Read the model definition and answer for the solid it produces. Units are mm, in the model's axes. Face numbers are marked on the shaded views. A direction names the side the tool comes from. Coordinates: 2 decimals unless noted, no trailing zeros. Order: outer loops, then holes, each group sorted by start corner. A loop starts at its lowest first (then second) coordinate and runs counter-clockwise, first axis right, second up. Notation, with made-up numbers: (89.5, -27.75) -> (135.5, -27.75) arc R18 cw to (135.5, -10.75) -> close; hole circle Ø5 at (-3.75, 21.5). An arc over 180 degrees is marked (long way). Use CSV: the item, a comma, the result in double quotes.
```python
from build123d import *

# Parameters (mm, degrees)
CROQUIS1_R              = 1.651
CROQUIS1_R_2            = 1.3208
SALIENTE_EXTRUIR1_DEPTH = 3.1242
CORTAR_EXTRUIR1_DEPTH   = 3.1242


with BuildPart() as part:
    # Croquis1 → Saliente-Extruir1 (new body)
    with BuildSketch(Plane.XY):
        with BuildLine():
            ThreePointArc((2.520278818, -2.298225244), (5.5245, -0.523415469), (8.528721182, -2.298225244))
            ThreePointArc((8.528721182, -2.298225244), (15.964986845, -3.467169905), (15.244404767, 4.025842847))
            ThreePointArc((15.244404767, 4.025842847), (7.556394525, 12.189930179), (4.7625, 23.0505))
            ThreePointArc((4.7625, 23.0505), (-0.866847253, 27.733445877), (-4.446941298, 21.345765609))
            ThreePointArc((-4.446941298, 21.345765609), (-3.013234987, 11.681947272), (-5.809588918, 2.321108456))
            ThreePointArc((-5.809588918, 2.321108456), (-3.960675565, -4.164949584), (2.520278818, -2.298225244))
        make_face()
        with Locations((-1.651, 0)):
            Circle(CROQUIS1_R, mode=Mode.SUBTRACT)
        Polygon((4.638514436, 4.7625), (3.464816339, 4.7625), (3.599843554, 6.647687651), align=None, mode=Mode.SUBTRACT)
        with Locations((0, 23.0505)):
            Circle(CROQUIS1_R_2, mode=Mode.SUBTRACT)
        with Locations((12.7, 0)):
            Circle(CROQUIS1_R, mode=Mode.SUBTRACT)
    extrude(amount=SALIENTE_EXTRUIR1_DEPTH)

    # Croquis2 → Cortar-Extruir1 (cut)
    with BuildSketch(Plane.XY.offset(3.1242)):
        with BuildLine():
            ThreePointArc((6.772401381, 2.38125), (7.178118311, 3.26217793), (7.753887726, 4.042645627))
            Line((7.753887726, 4.042645627), (2.361995667, 13.828929715))
            ThreePointArc((2.361995667, 13.828929715), (2.041810785, 13.746918232), (1.71670875, 13.687311946))
            Line((1.71670875, 13.687311946), (1.018825269, 3.943784893))
            ThreePointArc((1.018825269, 3.943784893), (1.834815442, 3.24507272), (2.473445986, 2.38125))
            Line((2.473445986, 2.38125), (6.772401381, 2.38125))
        make_face()
    extrude(amount=-CORTAR_EXTRUIR1_DEPTH, mode=Mode.SUBTRACT)


solid = part.part
```
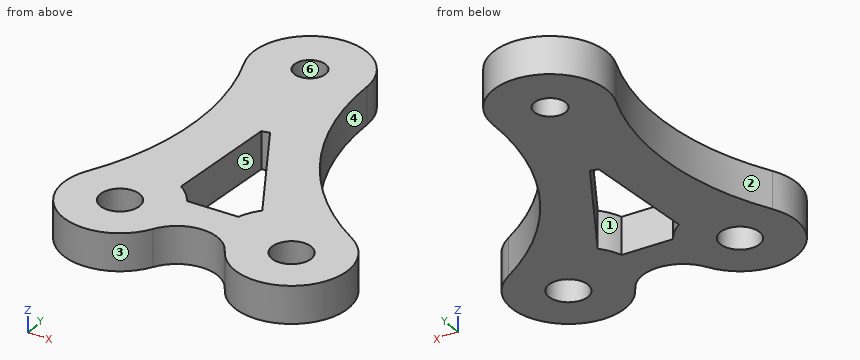
Item 1: The mould has two halves that part along Y. Classify the marked faces 3, 4, 5 and 6: +Y half, -Y half, draft (parallel to the pull), parting line (faces both ways), or undercut.
Return value:
face 3,"parting line"
face 4,"+Y half"
face 5,"undercut"
face 6,"undercut"
Item 2: A tool of negligible diameter and unlimited length cuts with its end or side. For the marked faces 1 and 2, from which of +Z, -Z, +X, -X, +Y, -Y can it reach the whole face along a straight path? Write none if from no direction.
Return value:
face 1,"+Z, -Z"
face 2,"+Z, -Z, -X"
Item 3: Find section D-D, the plane y = 20. Give the vertices of the cut face in (x, z), then the cut area to 3 significant figures.
Return value:
outline,"(-3.98, 0) -> (4.97, 0) -> (4.97, 3.12) -> (-3.98, 3.12) -> close"
area,"28.0 mm^2"
Item 4: Find section C-C, the plane z = 2.55. Give the vertices of the cut face in (x, y) (1 decimal), then the cut area to 3 significant figures.
Return value:
outline,"(-5.8, 2.3) arc R4.8 ccw to (2.5, -2.3) arc R3.4 cw to (8.5, -2.3) arc R4.8 ccw (long way) to (15.2, 4) arc R22.5 cw to (4.8, 23.1) arc R4.8 ccw (long way) to (-4.4, 21.3) arc R22.5 cw to start; hole circle Ø3.3 at (-1.7, 0); hole circle Ø2.6 at (0, 23.1); hole (1, 3.9) arc R4.8 cw to (2.5, 2.4) -> (6.8, 2.4) arc R4.8 cw to (7.8, 4) -> (2.4, 13.8) arc R4.8 cw to (1.7, 13.7) -> close; hole circle Ø3.3 at (12.7, 0)"
area,"353 mm^2"
Item 5: Find section A-A, the plane y = 0. Give the vertices of the cut face in (x, z).
Return value:
outline,"(-6.41, 0) -> (-3.3, 0) -> (-3.3, 3.12) -> (-6.41, 3.12) -> close; (0, 0) -> (11.05, 0) -> (11.05, 3.12) -> (0, 3.12) -> close; (14.35, 0) -> (17.46, 0) -> (17.46, 3.12) -> (14.35, 3.12) -> close"
Item 6: Find section B-B, the plane x = 12.25. Give the vertices of the cut face in (y, z), then the cut area to 3 significant figures.
Return value:
outline,"(-4.74, 0) -> (-1.59, 0) -> (-1.59, 3.12) -> (-4.74, 3.12) -> close; (1.59, 0) -> (6.29, 0) -> (6.29, 3.12) -> (1.59, 3.12) -> close"
area,"24.5 mm^2"
Item 7: Straight lines are drawn through the part: line 1 along X through (y, z) = (-1, 2.8); line 2 along Y through (x, z) = (-0.25, 0.4); line 3 along Y through (x, z) = (12.7, 0.8). For each, find the intervals that lie inside material, in ascending order.
Return value:
line 1,"x = -6.31 to -2.96, -0.34 to 3.78, 7.27 to 11.39, 14.01 to 17.36"
line 2,"y = -4.55 to -0.87, 0.87 to 21.75, 24.35 to 27.81"
line 3,"y = -4.76 to -1.65, 1.65 to 5.9"
